from build123d import *

# Parameters (mm, degrees)
F1_DEPTH       = 3.175
F2_R           = 6.35
F4_D           = 4.3
F4_CSINK_D     = 8
F4_CSINK_ANGLE = 90
F6_D           = 4
F6_CSINK_D     = 8
F6_CSINK_ANGLE = 90


with BuildPart() as f1:
    # F0 (on Top) → F1 (new body)
    with BuildSketch(Plane.XY):
        with BuildLine():
            Line((105.375, 0), (0, 0))
            Line((0, 0), (0, -93.225))
            Line((0, -93.225), (216.7, -93.225))
            Line((216.7, -93.225), (216.7, -42.525))
            Line((216.7, -42.525), (126.612, -42.525))
            Line((126.612, -42.525), (126.612, 0))
            Line((126.612, 0), (116.875, 0))
            Line((116.875, 0), (116.875, -34.25))
            ThreePointArc((116.875, -34.25), (111.125, -40), (105.375, -34.25))
            Line((105.375, -34.25), (105.375, 0))
        make_face()
    extrude(amount=F1_DEPTH)

    # F2
    f2_edges = [f1.edges().sort_by_distance(p)[0] for p in [
        (0, 0, 1.5875),
        (0, -93.225, 1.5875),
        (126.612, -42.525, 1.5875),
        (216.7, -42.525, 1.5875),
        (216.7, -93.225, 1.5875),
    ]]
    fillet(f2_edges, radius=F2_R)

    # F4 (through all)
    with Locations(Plane.XY.offset(3.175)):
        with Locations((5, -5), (5, -88.225), (211.7, -88.225), (211.7, -47.525), (136.612, -45.7), (83, -3.175), (108.35, -90.05)):
            CounterSinkHole(F4_D / 2, F4_CSINK_D / 2, counter_sink_angle=F4_CSINK_ANGLE)

    # F6 (through all)
    with Locations(Plane.XY.offset(3.175)):
        with Locations((123.437, -42.875), (123.437, -6.875), (93.262, -6.875), (93.262, -42.875)):
            CounterSinkHole(F6_D / 2, F6_CSINK_D / 2, counter_sink_angle=F6_CSINK_ANGLE)


solid = f1.part
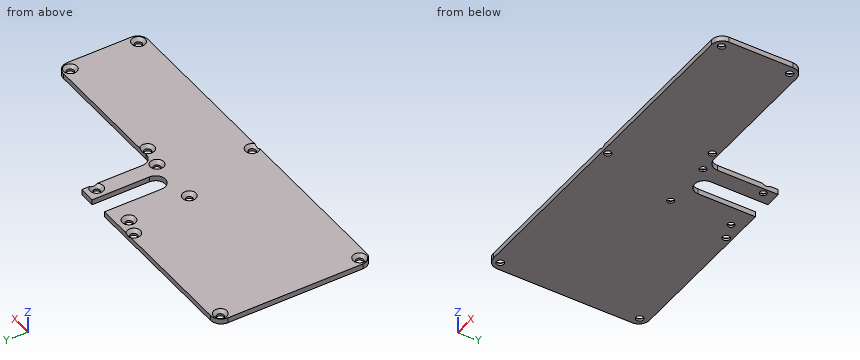
CAD build for the part. Positions are in the model's coordinates, mm. Round coordinates to 2 decimals unless told otherwise and drop trailing zeros. Write each loop counter-clockwise with the first axis right and the second up, starting at its lowest first coordinate (ties: lowest second). Pieces come first, ordered by that corner, then holes. Notation, with made-up numbers: (10.5, -36) -> (58.5, -36) arc R31 ccw to (58.5, -3) -> close; hole circle Ø11 at (-31, 9). An arc over 180 degrees is marked (long way). Answer as a JSON object with one key per item and string values.
(1) Band-saw the part on A-A, the plane y = -22.5. List the corners of the cut face in (x, z) (3 decimals), then the cut area to 3 significant figures.
Reported:
{"outline": "(0, 0) -> (105.375, 0) -> (105.375, 3.175) -> (0, 3.175) -> close; (116.875, 0) -> (126.612, 0) -> (126.612, 3.175) -> (116.875, 3.175) -> close", "area": "365 mm^2"}
(2) Band-saw the part on C-C, the plane z = 2.3. Count the separate pieces of the cut face and the enclosed holes in it, then the cut area to 3 significant figures.
Reported:
{"separate pieces": "1", "enclosed holes": "11", "area": "15,600 mm^2"}
(3) Pin check, flat tips, straight feed: P1, Ø3.5, axis at x = 5, y = -88.225, coming from the -Z side; P2, Ø5, axis at x = 123.437, y = -42.875, coming from the +Z side (3 decimals); P3, Ø5.5, axis at x = 211.7, y = -88.225, coming from the +Z side (3 decimals). Stop position of each tip, or through.
Reported:
{"P1": "passes through", "P2": "stops at z = 1.675", "P3": "stops at z = 1.925"}
(4) Band-saw the part on D-D, the plane x = 108.35. List the corners of the cut face in (y, z) (3 decimals), then the cut area to 3 significant figures.
Reported:
{"outline": "(-93.225, 0) -> (-92.2, 0) -> (-92.2, 1.325) -> (-93.225, 2.35) -> close; (-87.9, 0) -> (-39.286, 0) -> (-39.286, 3.175) -> (-86.05, 3.175) -> (-87.9, 1.325) -> close", "area": "155 mm^2"}
(5) Probe probe 1 along X at (y, z) = (-26.5, 2.15) (3 decimals); probe 2 along Y at (x, z) = (126, 2.75) (3 decimals); probe 3 along X at (y, z) = (-4, 0.9) (3 decimals). List the from-to ranges inside material, lowest first. Write a range as [from, to].
Reported:
{"probe 1": "x = [0, 105.375], [116.875, 126.612]", "probe 2": "y = [-93.225, -45.367], [-40.383, -9.367], [-4.383, 0]", "probe 3": "x = [0.451, 3.097], [6.903, 81.015], [84.985, 105.375], [116.875, 126.612]"}
(6) Band-saw the part on B-B, the plane x = 83. List the corners of the cut face in (y, z) (3 decimals).
Reported:
{"outline": "(-93.225, 0) -> (-5.325, 0) -> (-5.325, 1.325) -> (-7.175, 3.175) -> (-93.225, 3.175) -> close; (-1.025, 0) -> (0, 0) -> (0, 2.35) -> (-1.025, 1.325) -> close"}
